Part print with two shaded views. Sizes in mm from the minimum x, y, z corner. A direction names the side the tool comes from. Give positions to 0.01 mm unless a question says otherwise; leave off trailing zeros. Write each loop counter-clockwise with the first axis right and the second up, starting at its lowest first coordinate (ties: lowest second). Pieces come first, ordered by that corner, then holes. Notation, with made-up numbers: M -36,81.5 L -32,81.5 A20 cw -32,99.5 Z; hole C -10.5,81.25 d8. An arc over 180 degrees is marked long. One line per item, written item: value. Start each with the question number.
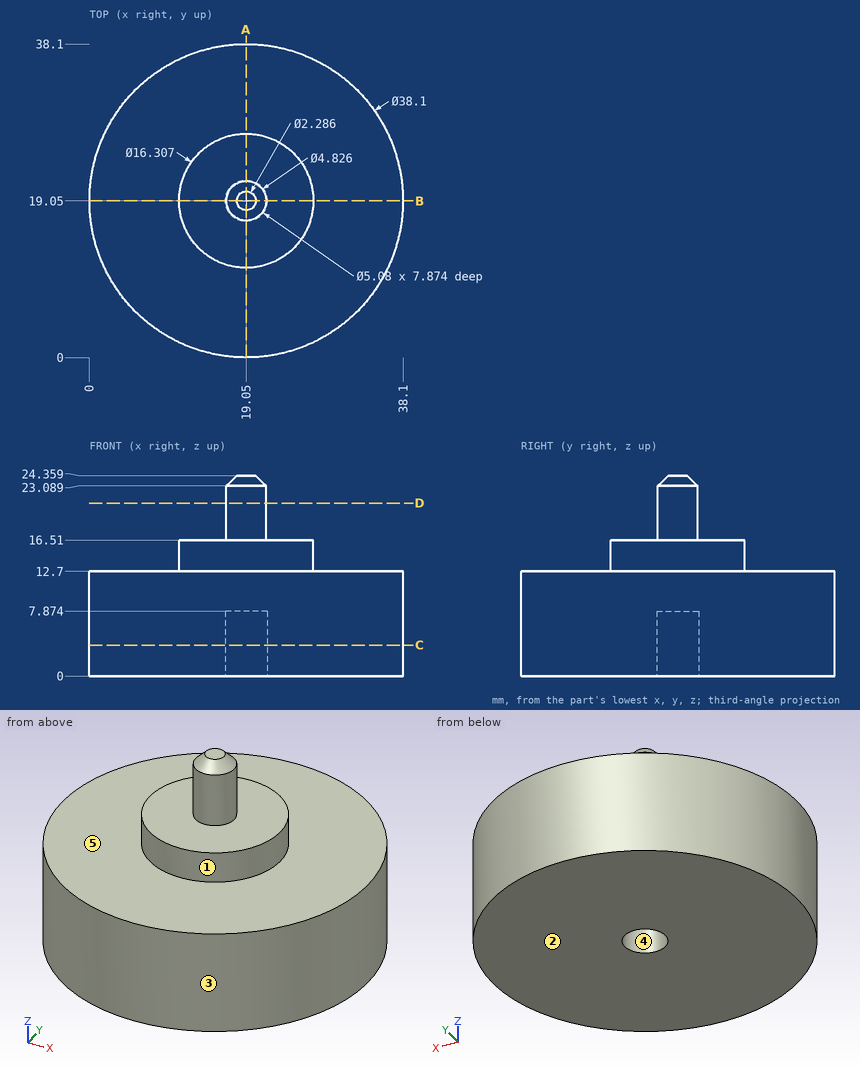
1) Band-saw the part on D-D (z = 21). List the corners of the cut face in (x, y).
2) Drop flat-ended pins along their axis: P1, Ø4, axis at x = 19, y = 19.5, coming from the -Z side; P2, Ø8, axis at x = 20, y = 16.5, coming from the +Z side; P3, Ø4, axis at x = 21, z = 4, coming from the +Y side; P4, Ø4, axis at x = 4.5, z = 5.5, coming from the -Y side. Give the stop position or say it passes through.
3) Mould opens along Y. For the marked faces 3, 4 and 5 say: released by +Y, released by -Y, zero draft, split by the parting line, or undercut.
4) Tool access for the marked faces 1 and 2: list every direction of +Z, -Z, +X, -X, +Y, -Y with a clear straight run to the whole face (end or side of a thin tool).
5) Band-saw the part on A-A (x = 19.05). List the corners of the cut face in (y, z).
6) Probe line 1 along Y through (x, z) = (19.05, 3.25); line 2 along Z through (x, y) = (24.5, 16). List the from-to ranges inside material, lowest first. Write a range as from..to.
7) Band-saw the part on C-C (z = 3.75). List the corners of the cut face in (x, y).
Model answer:
1. outline: C 19.05,19.05 d4.83
2. P1: stops at z = 7.87
2. P2: stops at z = 24.36
2. P3: stops at y = 38.1
2. P4: stops at y = 4.72
3. face 3: split by the parting line
3. face 4: undercut
3. face 5: zero draft
4. face 1: +Z
4. face 2: -Z, +X, -X, +Y, -Y
5. outline: M 0,0 L 16.51,0 L 16.51,7.87 L 21.59,7.87 L 21.59,0 L 38.1,0 L 38.1,12.7 L 27.2,12.7 L 27.2,16.51 L 21.46,16.51 L 21.46,23.09 L 20.19,24.36 L 17.91,24.36 L 16.64,23.09 L 16.64,16.51 L 10.9,16.51 L 10.9,12.7 L 0,12.7 Z
6. line 1: y = 0..16.51, 21.59..38.1
6. line 2: z = 0..16.51
7. outline: C 19.05,19.05 d38.1; hole C 19.05,19.05 d5.08
